For this review, use the dimensioned drawing (mm, ordinates from the lowest corner) and the shaded views. A direction names the side the tool comes from. Coordinates: 2 decimals unless noted, no trailing zeros. Loops run counter-clockwise (first coordinate to the right, second up) from the corner with the lowest first, then second, coordinate; pieces in that order, holes last. Notation, with made-up numbers: M -31.5,7.25 L -22.5,7.25 A34 cw -22.5,42.25 Z; hole C 10.25,86.25 d10. An arc over 180 degrees is marked long. One line per item, written item: value.
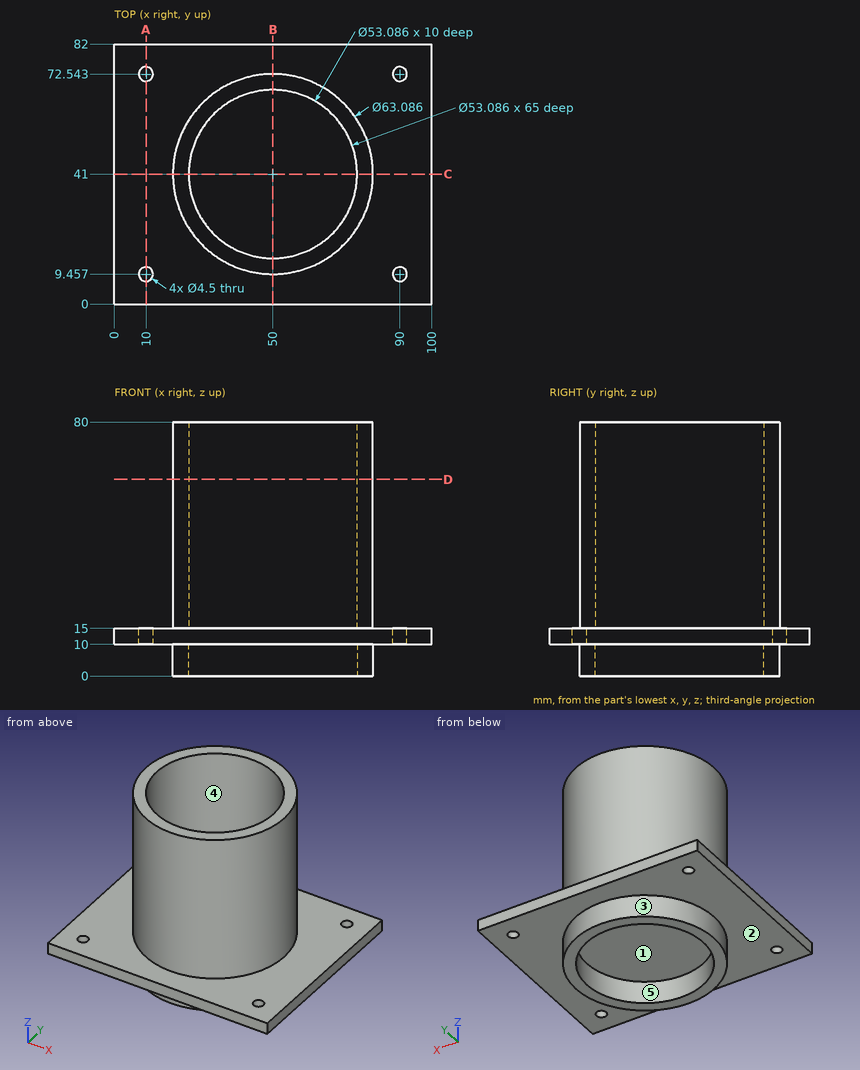
(1) Add section C-C on y = 41. State the section outline as (x, z) points, then the cut area to 3 significant figures.
Checks:
outline: M 0,10 L 18.46,10 L 18.46,0 L 23.46,0 L 23.46,10 L 76.54,10 L 76.54,0 L 81.54,0 L 81.54,10 L 100,10 L 100,15 L 81.54,15 L 81.54,80 L 76.54,80 L 76.54,15 L 23.46,15 L 23.46,80 L 18.46,80 L 18.46,15 L 0,15 Z
area: 1,250 mm^2
(2) Add section B-B on x = 50. State the section outline as (y, z) points.
Checks:
outline: M 0,10 L 9.46,10 L 9.46,0 L 14.46,0 L 14.46,10 L 67.54,10 L 67.54,0 L 72.54,0 L 72.54,10 L 82,10 L 82,15 L 72.54,15 L 72.54,80 L 67.54,80 L 67.54,15 L 14.46,15 L 14.46,80 L 9.46,80 L 9.46,15 L 0,15 Z
(3) Add section D-D on z = 62. State the section outline as (x, y) points.
Checks:
outline: C 50,41 d63.09; hole C 50,41 d53.09
(4) Draft analysis for pull direction X (two halves, no side actions). For the marked faces 1, 2 and 3, state which applies: pulls with the +X half, pulls with the -X half, needs draft (parallel to the pull), parting line crosses it, or undercut.
Checks:
face 1: undercut
face 2: needs draft
face 3: parting line crosses it
(5) Add section A-A on x = 10. State the section outline as (y, z) points.
Checks:
outline: M 0,10 L 7.21,10 L 7.21,15 L 0,15 Z; M 11.71,10 L 70.29,10 L 70.29,15 L 11.71,15 Z; M 74.79,10 L 82,10 L 82,15 L 74.79,15 Z
(6) Tool access review of the marked faces 4 and 5: name each direction out of +Z, -Z, +X, -X, +Y, -Y from which nothing blocks a thin tool from reaching the whole face with its end or side.
Checks:
face 4: +Z
face 5: -Z
(7) To check wall thickness, follow L1, parallel to Y at x = 10, z = 13; L2, parallel to X at y = 11.5, z = 14.5; L3, parallel to X at y = 40.5, z = 35. State the ranges of each line that lie inside material, in increasing order. Write a range as [from, to].
Checks:
L1: [0, 7.21], [11.71, 70.29], [74.79, 82]
L2: [0, 9.06], [10.94, 89.06], [90.94, 100]
L3: [18.46, 23.46], [76.54, 81.54]
(8) Insertion check: pin 1 Ø6 at (x, z) = (30.5, 50.5) entering from +Y; pin 2 Ø6 at (x, y) = (10, 9.457) entering from +Z; pin 3 Ø1 at (x, z) = (56.5, 19) entering from +Y. Each pin has a flat end and moves straight along its axis. Give the tip position at first contact, or say it passes through.
Checks:
pin 1: y = 67.88
pin 2: z = 15
pin 3: y = 71.97
